Source: CAD feature listing. Evaluate the final solid. Frame: model axes, mm. A direction names the side the tool comes from. Give positions to 0.01 mm unless a question says otherwise; leave off trailing zeros. Write each loop counter-clockwise with the first axis right and the second up, starting at its lowest first coordinate (ties: lowest second). Pieces come first, ordered by that corner, then holes. Notation, with made-up numbers: (-4, 77.5) - (15, 77.5) arc R38 cw to (15, 115.5) - close; hole circle Ø1 at (44, 68.5). An arc over 180 degrees is marked (long way). Answer as a JSON object with one key per item and string values. Group by question number.
from build123d import *

# Parameters (mm, degrees)
F1_DEPTH = 19.05
F0_W     = 19.05
F0_H     = 19.05
F2_DEPTH = 38.1
F3_DEPTH = 19.05


with BuildPart() as f1:
    # F0 (on Top) → F1 (new body)
    with BuildSketch(Plane.XY):
        Polygon((17.895463, -38.1), (0, -38.1), (-19.05, -38.1), (-19.05, -57.15), (17.895463, -57.15), align=None)
    extrude(amount=F1_DEPTH)

    # F0 (on Top) → F2 (join)
    with BuildSketch(Plane.XY):
        with Locations((-9.525, -28.575)):
            Rectangle(F0_W, F0_H)
    extrude(amount=F2_DEPTH)

    # F0 (on Top) → F3 (join)
    with BuildSketch(Plane.XY):
        with Locations((-9.525, -9.525)):
            Rectangle(F0_W, F0_H)
    extrude(amount=F3_DEPTH)


solid = f1.part
Q1. First-contact query: pin 1 Ø5 at (x, z) = (8, 24) entering from -Y; pin 2 Ø5.5 at (x, z) = (-5, 31) entering from -Y; pin 3 Ø9.5 at (x, y) = (-13.5, -6) entering from +Z; pin 4 Ø4 at (x, z) = (1.5, 32.5) entering from +Y. Flat tips, straight axial feed; report the tip coordinate or a pass-through.
Q2. Section B-B on y = -6. Return the cut outline in (x, z).
Q3. Section C-C on z = 11. Return the cut outline in (x, y), then the cut area to 3 significant figures.
Q4. Ray query, probe 1 along Y at (x, z) = (13, 18.5); probe 2 along X at (y, z) = (-9, 11.5); probe 3 along Z at (x, y) = (-14, -44.5). Return the intervals inside material, ascending. Write a range as [from, to].
Q5. Section A-A on x = -7.5. Return the cut outline in (y, z).
Q6. Reachability of faces 1 (the flat face through (0, -24, 15)), 2 (the flat face through (-1, -47, 19.05)), 3 (the flat face through (-10, -19.05, 28)) from +Z, -Z, +X, -X, +Y, -Y: full face, straight path, thin tool, end or side. Return the list, or none.
Q7. Section D-D on y = -44.5. Return the cut outline in (x, z), then the cut area to 3 significant figures.
Taken from the geometry:
{
 "1": {"pin 1": "passes through", "pin 2": "stops at y = -38.1", "pin 3": "stops at z = 19.05", "pin 4": "stops at y = -19.05"},
 "2": {"outline": "(-19.05, 0) - (0, 0) - (0, 19.05) - (-19.05, 19.05) - close"},
 "3": {"outline": "(-19.05, -57.15) - (17.9, -57.15) - (17.9, -38.1) - (0, -38.1) - (0, 0) - (-19.05, 0) - close", "area": "1,430 mm²"},
 "4": {"probe 1": "y = [-57.15, -38.1]", "probe 2": "x = [-19.05, 0]", "probe 3": "z = [0, 19.05]"},
 "5": {"outline": "(-57.15, 0) - (0, 0) - (0, 19.05) - (-19.05, 19.05) - (-19.05, 38.1) - (-38.1, 38.1) - (-38.1, 19.05) - (-57.15, 19.05) - close"},
 "6": {"face 1": "+Z, -Z, +X, +Y", "face 2": "+Z, +X, -X, -Y", "face 3": "+Z, +X, -X, +Y"},
 "7": {"outline": "(-19.05, 0) - (17.9, 0) - (17.9, 19.05) - (-19.05, 19.05) - close", "area": "704 mm²"}
}
